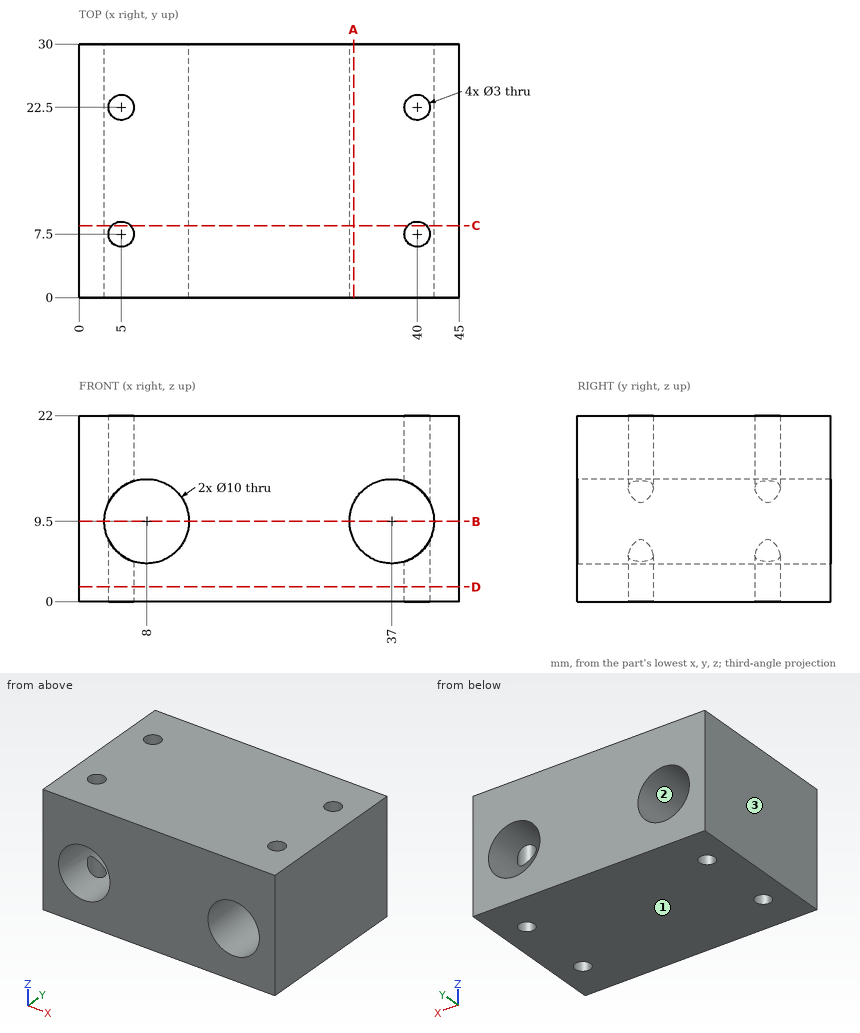
Verification items for this drawing (mm, ordinates from the low corner). Give positions to 0.01 mm unless a question says otherwise; leave off trailing zeros. Write each loop counter-clockwise with the first axis right and the second up, starting at its lowest first coordinate (ties: lowest second). Pieces come first, ordered by that corner, then holes. Notation, with made-up numbers: (11.25, 77.25) -> (27.25, 77.25) arc R15 ccw to (27.25, 94.25) -> close; hole circle Ø9 at (-4.75, -3.75). An arc over 180 degrees is marked (long way). Use CSV: the item, a comma, the result in double quotes.
(1) Release check for a two-part mould opening along Z. For the marked faces 1, 2 and 3 record: +Z half, -Z half, draft (parallel to the pull), parting line (faces both ways), or undercut.
Derived:
face 1,"-Z half"
face 2,"undercut"
face 3,"draft"
(2) Sectioned sample at B-B (z = 9.5). Record the cut outline in (x, y), plus the area to 3 significant figures.
Derived:
outline,"(0, 0) -> (3, 0) -> (3, 30) -> (0, 30) -> close; (13, 0) -> (32, 0) -> (32, 30) -> (13, 30) -> close; (42, 0) -> (45, 0) -> (45, 30) -> (42, 30) -> close"
area,"750 mm^2"
(3) Sectioned sample at D-D (z = 1.75). Record the cut outline in (x, y).
Derived:
outline,"(0, 0) -> (45, 0) -> (45, 30) -> (0, 30) -> close; hole circle Ø3 at (5, 7.5); hole circle Ø3 at (5, 22.5); hole circle Ø3 at (40, 7.5); hole circle Ø3 at (40, 22.5)"
(4) Sectioned sample at C-C (y = 8.5). Record the cut outline in (x, z).
Derived:
outline,"(0, 0) -> (3.88, 0) -> (3.88, 6.66) arc R5 cw to (3.88, 12.34) -> (3.88, 22) -> (0, 22) -> close; (6.12, 0) -> (38.88, 0) -> (38.88, 4.87) arc R5 cw (long way) to (38.88, 14.13) -> (38.88, 22) -> (6.12, 22) -> (6.12, 14.13) arc R5 cw (long way) to (6.12, 4.87) -> close; (41.12, 0) -> (45, 0) -> (45, 22) -> (41.12, 22) -> (41.12, 12.34) arc R5 cw to (41.12, 6.66) -> close"
(5) Material ranges on L1, parallel to Y at x = 40, z = 15.75; L2, parallel to X at y = 7, z = 17.5; L3, parallel to Z at x = 4, y = 16, recorded low to high.
Derived:
L1,"y = 0 to 6, 9 to 21, 24 to 30"
L2,"x = 0 to 3.59, 6.41 to 38.59, 41.41 to 45"
L3,"z = 0 to 6.5, 12.5 to 22"
(6) Sectioned sample at A-A (x = 32.5). Record the cut outline in (y, z), plus the area to 3 significant figures.
Derived:
outline,"(0, 0) -> (30, 0) -> (30, 7.32) -> (0, 7.32) -> close; (0, 11.68) -> (30, 11.68) -> (30, 22) -> (0, 22) -> close"
area,"529 mm^2"
